Job drawing, mm, ordinate dimensions from the low corner. One solid piece. Round coordinates to 2 decimals unless told otherwise and drop trailing zeros. Write each loop counter-clockwise with the first axis right and the second up, starting at its lowest first coordinate (ties: lowest second). Pieces come first, ordered by that corner, then holes.
1) Saw through at C-C (y = 6). Write the cut outline in (x, z).
2) Saw through at B-B (x = 0.2). Write the cut outline in (y, z), plus the area to 3 significant figures.
3) Wall check: probe 1 along Y at (x, z) = (0.1, 4); probe 2 along Z at (x, y) = (0.2, 14); probe 3 along Z at (x, y) = (0.25, 15.5). Give the ranges that are in metal, low to high.
4) Saw through at A-A (z = 4). Write the cut outline in (x, y), plus the area to 3 significant figures.
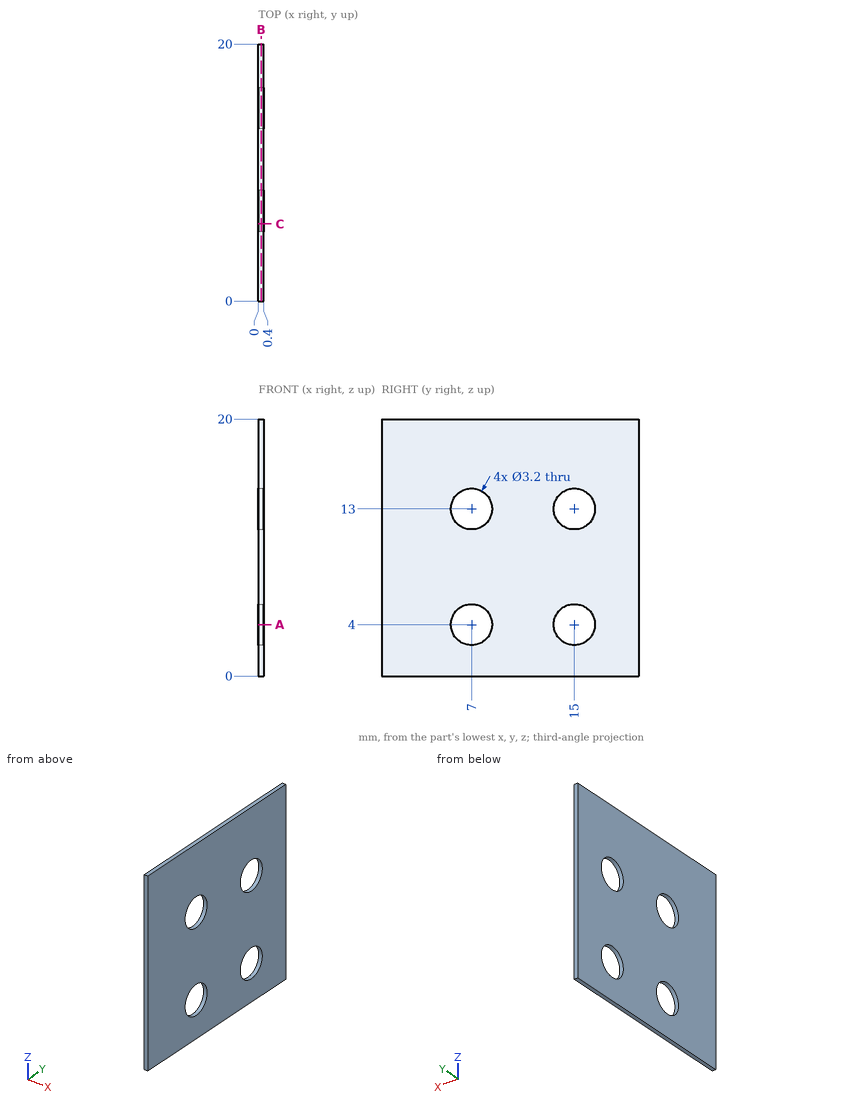
Evaluation:
1. outline: (0, 0) - (0.4, 0) - (0.4, 2.75) - (0, 2.75) - close; (0, 5.25) - (0.4, 5.25) - (0.4, 11.75) - (0, 11.75) - close; (0, 14.25) - (0.4, 14.25) - (0.4, 20) - (0, 20) - close
2. outline: (0, 0) - (20, 0) - (20, 20) - (0, 20) - close; hole circle Ø3.2 at (7, 4); hole circle Ø3.2 at (7, 13); hole circle Ø3.2 at (15, 4); hole circle Ø3.2 at (15, 13)
2. area: 368 mm2
3. probe 1: y = 0 to 5.4, 8.6 to 13.4, 16.6 to 20
3. probe 2: z = 0 to 2.75, 5.25 to 11.75, 14.25 to 20
3. probe 3: z = 0 to 2.48, 5.52 to 11.48, 14.52 to 20
4. outline: (0, 0) - (0.4, 0) - (0.4, 5.4) - (0, 5.4) - close; (0, 8.6) - (0.4, 8.6) - (0.4, 13.4) - (0, 13.4) - close; (0, 16.6) - (0.4, 16.6) - (0.4, 20) - (0, 20) - close
4. area: 5.44 mm2
